```python
from build123d import *

# Parameters (mm, degrees)
SKETCH2_W           = 30.751006124
SKETCH2_H           = 0.5
SKETCH2_W_2         = 3.100075991
SKETCH2_H_2         = 10.000695173
SKETCH2_W_3         = 2
SKETCH2_H_3         = 3.50017022
SKETCH2_W_4         = 1.95
BOSS_EXTRUDE1_DEPTH = 2
SKETCH3_W           = 1.150075991
SKETCH3_H           = 6.000695173
SKETCH3_W_2         = 1.100075991
BOSS_EXTRUDE2_DEPTH = 1.5
SKETCH4_W           = 1.550075991
SKETCH4_H           = 4.899134607
SKETCH4_H_2         = 6.400695173
SKETCH4_W_2         = 1.500075991
BOSS_EXTRUDE3_DEPTH = 1
CHAMFER1_SIZE       = 0.2
CUT_EXTRUDE1_START  = -2
SKETCH5_W           = 3.300200616
SKETCH5_H           = 1
SKETCH5_W_2         = 3.300200617
CUT_EXTRUDE1_DEPTH  = 2
SKETCH8_W           = 16.850185419
SKETCH8_H           = 0.5
BOSS_EXTRUDE4_DEPTH = 2
CHAMFER2_SIZE       = 2


with BuildPart() as part:
    # Sketch2 → Boss-Extrude1 (new body)
    with BuildSketch(Plane.XY):
        Polygon((277.431409328, 90.45473243), (281.431409328, 90.45473243), (281.431409328, 91.95473243), (262.955830275, 91.95473243), (262.955830275, 84.955597823), (264.905830275, 84.955597823), (266.055906266, 84.955597823), (266.055906266, 87.985794184), (273.006316619, 87.985794184), (273.006316619, 84.955597823), (274.331409328, 84.955597823), (274.331409328, 89.55473243), (277.431409328, 89.55473243), align=None)
        Polygon((281.431409328, 91.95473243), (281.431409328, 90.45473243), (285.431409328, 90.45473243), (285.431409328, 89.55473243), (288.531409328, 89.55473243), (288.531409328, 84.955597823), (289.856502038, 84.955597823), (289.856502038, 87.985794184), (296.80691239, 87.985794184), (296.80691239, 84.955597823), (297.906988381, 84.955597823), (299.906988381, 84.955597823), (299.906988381, 91.95473243), align=None)
        with Locations((281.431409328, 71.70473243)):
            Rectangle(SKETCH2_W, SKETCH2_H)
        with Locations((264.505868271, 76.455080017)):
            Rectangle(SKETCH2_W_2, SKETCH2_H_2)
        Polygon((299.906988381, 71.45473243), (299.906988381, 81.455427603), (297.906988381, 81.455427603), (296.80691239, 81.455427603), (296.80691239, 71.95473243), (296.80691239, 71.45473243), align=None)
        with Locations((298.906988381, 83.205512713)):
            Rectangle(SKETCH2_W_3, SKETCH2_H_3)
        with Locations((263.930830275, 83.205512713)):
            Rectangle(SKETCH2_W_4, SKETCH2_H_3)
    extrude(amount=-BOSS_EXTRUDE1_DEPTH)

    # Sketch3 → Boss-Extrude2 (add)
    with BuildSketch(Plane.XY):
        Polygon((265.005830275, 84.955597823), (266.055906266, 84.955597823), (266.055906266, 87.985794184), (273.006316619, 87.985794184), (273.006316619, 84.955597823), (274.331409328, 84.955597823), (274.331409328, 89.45473243), (265.005830275, 89.45473243), align=None)
        with Locations((265.480868271, 78.455080017)):
            Rectangle(SKETCH3_W, SKETCH3_H)
        with Locations((297.356950385, 78.455080017)):
            Rectangle(SKETCH3_W_2, SKETCH3_H)
        Polygon((288.531409328, 89.45473243), (288.531409328, 84.955597823), (289.856502038, 84.955597823), (289.856502038, 87.985794184), (296.80691239, 87.985794184), (296.80691239, 84.955597823), (297.856988381, 84.955597823), (297.856988381, 89.45473243), align=None)
    extrude(amount=BOSS_EXTRUDE2_DEPTH)

    # Sketch4 → Boss-Extrude3 (add)
    with BuildSketch(Plane.XY.offset(1.5)):
        with Locations((265.280868271, 87.405165127)):
            Rectangle(SKETCH4_W, SKETCH4_H)
        with Locations((265.280868271, 78.255080017)):
            Rectangle(SKETCH4_W, SKETCH4_H_2)
        with Locations((297.556950386, 78.255080017)):
            Rectangle(SKETCH4_W_2, SKETCH4_H_2)
        with Locations((297.581950386, 87.405165127)):
            Rectangle(SKETCH4_W, SKETCH4_H)
    extrude(amount=BOSS_EXTRUDE3_DEPTH)

    # Chamfer1
    chamfer1_edges = [part.edges().sort_by_distance(p)[0] for p in [
        (298.356988381, 87.405165127, 1.5),
        (297.581950386, 89.85473243, 1.5),
        (297.556950386, 75.05473243, 1.5),
        (298.306988381, 78.255080016, 1.5),
        (265.280868271, 75.05473243, 1.5),
        (264.505830275, 78.255080016, 1.5),
        (265.280868271, 89.85473243, 1.5),
        (264.505830275, 87.405165127, 1.5),
    ]]
    chamfer(chamfer1_edges, length=CHAMFER1_SIZE)

    # Sketch5 → Cut-Extrude1 (cut)
    with BuildSketch(Plane(origin=(0, 0, -2), x_dir=(-1, 0, 0), z_dir=(0, 0, -1)).offset(CUT_EXTRUDE1_START)):
        with Locations((-269.530111382, 88.485794184)):
            Rectangle(SKETCH5_W, SKETCH5_H)
        with Locations((-293.332707275, 88.485794184)):
            Rectangle(SKETCH5_W_2, SKETCH5_H)
    extrude(amount=CUT_EXTRUDE1_DEPTH, mode=Mode.SUBTRACT)

    # Sketch8 → Boss-Extrude4 (add)
    with BuildSketch(Plane(origin=(0, 0, -2), x_dir=(-1, 0, 0), z_dir=(0, 0, -1))):
        with Locations((-281.431409329, 72.20473243)):
            Rectangle(SKETCH8_W, SKETCH8_H)
    extrude(amount=-BOSS_EXTRUDE4_DEPTH)

    # Chamfer2
    chamfer2_edges = [part.edges().sort_by_distance(p)[0] for p in [
        (262.955830275, 91.95473243, -1),
        (299.906988381, 91.95473243, -1),
        (262.955830275, 71.45473243, -1),
        (299.906988381, 71.45473243, -1),
    ]]
    chamfer(chamfer2_edges, length=CHAMFER2_SIZE)


solid = part.part
```
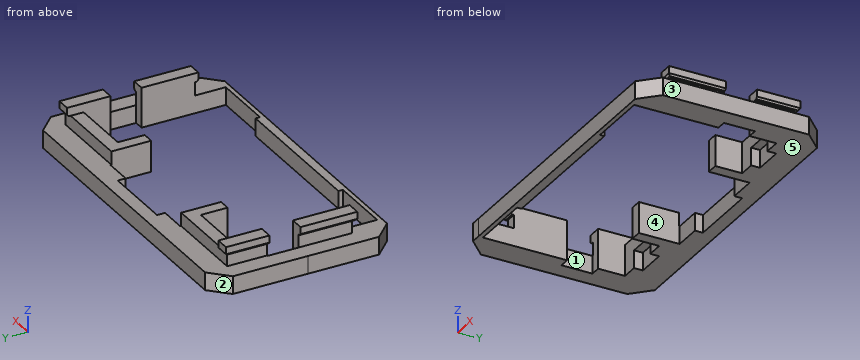
Check sheet for the modelled part. Datum: model origin and axes. Units: mm. Face numbers are marked on the shaded views. A direction names the side the tool comes from. Coordinates: 2 decimals unless noted, no trailing zeros. Order: outer loops, then holes, each group sorted by start corner. A loop starts at its lowest first (then second) coordinate and runs counter-clockwise, first axis right, second up. Notation, with made-up numbers: M 47,80 L 74,80 A15 ccw 74,90 Z; hole C -31,-31 d5. An arc over 180 degrees is marked long. One line per question, with ' | ' between items. Start each with the question number.
Item 1: Gauge pin test, flat ends, axial feed: P1, Ø0.8, axis at x = 298, z = 1.5, coming from the -Y side; P2, Ø10, axis at x = 280.5, y = 80.5, coming from the -Z side; P3, Ø0.9, axis at y = 88, z = 2.5, coming from the -X side. Record the tip position at first contact, or that the pin passes through.
Item 2: Sectioned sample at A-A on x = 287.5. Record the cut outline in (y, z), and give its area (3 significant figures).
Item 3: Sectioned sample at B-B on z = 1.05. Record the cut outline in (x, y), and give its area (3 significant figures).
Item 4: Material ranges on line 1 (X direction, y = 87, z = 1.2); line 2 (X direction, y = 86.5, z = 2.1); line 3 (Y direction, x = 266, z = 0.3), recorded low to high.
Item 5: Sectioned sample at C-C on y = 74.5. Record the cut outline in (x, z).
Item 6: Sectioned sample at D-D on x = 270. Record the cut outline in (y, z).
Item 7: Access from +Z, -Z, +X, -X, +Y, -Y to the whole of each face (thin tool, end or side, straight path). Record for the marked faces 4 and 5.
Item 8: Mould release check, pull along Y, two halves, no side actions. Record for the marked faces 1, 2 and 3: pulls with the +Y half, pulls with the -Y half, needs draft (parallel to the pull), parting line crosses it, or undercut.
Answer below:
1) P1: stops at y = 75.05 | P2: passes through | P3: stops at x = 264.51
2) outline: M 71.45,-2 L 72.45,-2 L 72.45,0 L 71.45,0 Z; M 89.55,-2 L 91.95,-2 L 91.95,0 L 89.55,0 Z | area: 6.80 mm^2
3) outline: M 264.91,75.45 L 266.06,75.45 L 266.06,81.46 L 264.91,81.46 Z; M 265.01,84.96 L 266.06,84.96 L 266.06,87.99 L 273.01,87.99 L 273.01,84.96 L 274.33,84.96 L 274.33,89.45 L 265.01,89.45 Z; M 288.53,84.96 L 289.86,84.96 L 289.86,87.99 L 296.81,87.99 L 296.81,84.96 L 297.86,84.96 L 297.86,89.45 L 288.53,89.45 Z; M 296.81,75.45 L 297.91,75.45 L 297.91,81.46 L 296.81,81.46 Z | area: 55.3 mm^2
4) line 1: x = 265.01 to 266.06, 273.01 to 274.33, 288.53 to 289.86, 296.81 to 297.86 | line 2: x = 264.51 to 266.06, 296.81 to 298.36 | line 3: y = 75.45 to 81.46, 84.96 to 89.45
5) outline: M 262.96,-2 L 266.06,-2 L 266.06,0 L 262.96,0 Z; M 296.81,-2 L 299.91,-2 L 299.91,0 L 296.81,0 Z
6) outline: M 71.45,-2 L 71.95,-2 L 71.95,0 L 71.45,0 Z; M 87.99,0 L 88.99,0 L 88.99,-2 L 91.95,-2 L 91.95,0 L 89.45,0 L 89.45,1.5 L 87.99,1.5 Z
7) face 4: +Z, -Z | face 5: -Z, +X, -X, +Y, -Y
8) face 1: undercut | face 2: pulls with the +Y half | face 3: needs draft
